Design review of the part built by this model. Coordinates are the model's own, in mm. A direction names the side the tool comes from. Round coordinates to 2 decimals unless told otherwise and drop trailing zeros. Loops run counter-clockwise (first coordinate to the right, second up) from the corner with the lowest first, then second, coordinate; pieces in that order, holes last. Notation, with made-up numbers: (47, 64.25) -> (96, 64.25) arc R21 ccw to (96, 79.25) -> close; hole circle Ø3 at (-32.5, 88.25). An arc over 180 degrees is marked (long way). Answer as CSV lines item,"result". Start each with the question number.
```python
from build123d import *

# Parameters (mm, degrees)
F1_DEPTH = 15.875


with BuildPart() as f1:
    # F0 (on Top) → F1 (new body)
    with BuildSketch(Plane.XY):
        with BuildLine():
            Line((88.9, 0), (3.420675, 0))
            ThreePointArc((3.420675, 0), (1.093601, -1.015058), (0.254473, -3.411196))
            Line((0.254473, -3.411196), (3.354198, -44.962916))
            ThreePointArc((3.354198, -44.962916), (4.360458, -47.053794), (6.5204, -47.901719))
            ThreePointArc((6.5204, -47.901719), (8.861255, -46.871718), (9.683318, -44.45))
            Line((9.683318, -44.45), (6.500993, -8.07586))
            ThreePointArc((6.500993, -8.07586), (6.912024, -6.865001), (8.082452, -6.35))
            Line((8.082452, -6.35), (84.1375, -6.35))
            ThreePointArc((84.1375, -6.35), (85.260032, -6.814968), (85.725, -7.9375))
            Line((85.725, -7.9375), (85.725, -95.25))
            ThreePointArc((85.725, -95.25), (104.775, -114.3), (123.825, -95.25))
            ThreePointArc((123.825, -95.25), (120.65, -92.075), (117.475, -95.25))
            ThreePointArc((117.475, -95.25), (104.775, -107.95), (92.075, -95.25))
            Line((92.075, -95.25), (92.075, -45.949032))
            ThreePointArc((92.075, -45.949032), (112.55213, -49.140191), (123.825, -31.75))
            ThreePointArc((123.825, -31.75), (120.65, -28.575), (117.475, -31.75))
            ThreePointArc((117.475, -31.75), (104.775, -44.45), (92.075, -31.75))
            Line((92.075, -31.75), (92.075, -3.175))
            ThreePointArc((92.075, -3.175), (91.145064, -0.929936), (88.9, 0))
        make_face()
    extrude(amount=F1_DEPTH)


solid = f1.part
```
Q1. Add section A-A, the plane x = 120.65. Give the boundary of the cut face in (y, z) (3 decimals).
Q2. Add section B-B, the plane y = -93.5. Give the boundary of the cut face in (x, z) (3 decimals).
Q3. To check wall thickness, follow probe 1 along Y at (x, z) = (105.5, 12.5); probe 2 along X at (y, z) = (-33.5, 4.75) (3 decimals); probe 3 along X at (y, z) = (-38.5, 11.25) (3 decimals). State the ranges of each line that lie inside material, in increasing order. Write a range as from..to.
Q4. Mouldability with a two-part tool opening along X and no side actions: class faces 4 (the flat face through (1.783, -23.896, 7.826)), 5 (the cylindrical face through (105.054, -44.447, 7.826)), 6 (the flat face through (89, -36, 0)) as pulls with the +X half, pulls with the -X half, needs draft (parallel to the pull), parting line crosses it, or undercut.
Q5. Machinability: for faces 1 (the flat face through (92.075, -71, 8)), 2 (the cylindrical face through (91.17, -0.955, 7.826)), 3 (the flat face through (85.725, -51, 8)), which of the approach directions +Z, -Z, +X, -X, +Y, -Y give a long, thin tool a straight path to every point of the face, cutting with its end or side? Answer none if there is none.
Q6. Add section D-D, the plane y = -61. Give the boundary of the cut face in (x, z) (3 decimals), and give its area (3 significant figures).
Q7. For pin 1 Ø2 at (y, z) = (-46, 12.5) entering from -X; pin 2 Ø5 at (x, z) = (26.5, 13.5) entering from -Y; pin 3 Ø10 at (x, y) = (80, -101.5) entering from -Z; pin 4 Ø5 at (y, z) = (-43, 6.5) entering from -X, all flat-tipped, find the tip position at first contact; note any pin that passes through.
Worked answers:
1,outline,"(-105.78, 0) -> (-92.075, 0) -> (-92.075, 15.875) -> (-105.78, 15.875) -> close; (-42.28, 0) -> (-28.575, 0) -> (-28.575, 15.875) -> (-42.28, 15.875) -> close"
2,outline,"(85.725, 0) -> (92.075, 0) -> (92.075, 15.875) -> (85.725, 15.875) -> close; (118.001, 0) -> (123.299, 0) -> (123.299, 15.875) -> (118.001, 15.875) -> close"
3,probe 1,"y = -114.29..-107.93, -50.79..-44.43"
3,probe 2,"x = 2.499..8.725, 85.725..92.196, 117.354..123.744"
3,probe 3,"x = 2.872..9.163, 85.725..94.017, 115.533..122.589"
4,face 4,"pulls with the -X half"
4,face 5,"undercut"
4,face 6,"needs draft"
5,face 1,"+Z, -Z"
5,face 2,"+Z, -Z, +X, +Y"
5,face 3,"+Z, -Z, -Y"
6,outline,"(85.725, 0) -> (92.075, 0) -> (92.075, 15.875) -> (85.725, 15.875) -> close"
6,area,"101 mm^2"
7,pin 1,"stops at x = 3.36"
7,pin 2,"stops at y = -6.35"
7,pin 3,"passes through"
7,pin 4,"stops at x = 3.02"
